Build history of the part. All positions in model axes, mm. A direction names the side the tool comes from. Give positions to 0.01 mm unless a question says otherwise; leave off trailing zeros. Order: outer loops, then holes, each group sorted by start corner. A loop starts at its lowest first (then second) coordinate and runs counter-clockwise, first axis right, second up. Notation, with made-up numbers: (-21.5, 28) - (-3.5, 28) arc R18 ccw to (-3.5, 52) - close; hole circle Ø4 at (-26, 36.5). An arc over 180 degrees is marked (long way). Answer in a Markdown table with one row per item.
```python
from build123d import *

# Parameters (mm, degrees)
F0_W      = 80
F0_H      = 40
F1_DEPTH  = 3
F2_R      = 3
F3_DEPTH  = 3
F5_D      = 2.5
F7_DEPTH  = 3
F9_D      = 3.25
F10_W     = 44.45
F10_H     = 19.05
F11_DEPTH = 6.001
F12_R     = 3
F13_R     = 1


# Not quite as in the source:
# - a pattern or mirror of a feature is missing from the dataset's text; its kind, count and spacing are read off the source's solid
# - a feature names something its author has since deleted; it is built from what else it names


with BuildPart() as f1:
    # F0 (on Top) → F1 (new body)
    with BuildSketch(Plane.XY):
        Rectangle(F0_W, F0_H)
    extrude(amount=F1_DEPTH)

    # F2 (on face) → F3 (join)
    with BuildSketch(Plane.XY.offset(3)):
        with Locations((-29, 11.5)):
            Circle(F2_R)
        with Locations((29, 11.5)):
            Circle(F2_R)
        with Locations((29, -11.5)):
            Circle(F2_R)
        with Locations((-29, -11.5)):
            Circle(F2_R)
    extrude(amount=F3_DEPTH)

    # F5 (through all)
    with Locations(Plane.XY.offset(6)):
        with Locations((-29, 11.5), (29, 11.5), (29, -11.5), (-29, -11.5)):
            Hole(F5_D / 2)

    # F6 (on face) → F7 (join)
    with BuildSketch(Plane(origin=(0, 0, 0), x_dir=(1, 0, 0), z_dir=(0, 0, -1))):
        with BuildLine():
            ThreePointArc((42.1213203436, 17.8786796564), (42.7716385975, 18.8519497029), (43, 20))
            ThreePointArc((43, 20), (41.1480502971, 22.7716385975), (37.8786796564, 22.1213203436))
            ThreePointArc((37.8786796564, 22.1213203436), (37.2283614025, 21.1480502971), (37, 20))
            Line((37, 20), (40, 20))
            Line((40, 20), (40, 17))
            ThreePointArc((40, 17), (41.1480502971, 17.2283614025), (42.1213203436, 17.8786796564))
        make_face()
        with BuildLine():
            ThreePointArc((37, 20), (37.2283614025, 21.1480502971), (37.8786796564, 22.1213203436))
            Line((37.8786796564, 22.1213203436), (35.7573593129, 20))
            Line((35.7573593129, 20), (37, 20))
        make_face()
        with BuildLine():
            Line((40, 15.7573593129), (42.1213203436, 17.8786796564))
            ThreePointArc((42.1213203436, 17.8786796564), (41.1480502971, 17.2283614025), (40, 17))
            Line((40, 17), (40, 15.7573593129))
        make_face()
        with BuildLine():
            Line((-37, 20), (-35.7573593129, 20))
            Line((-35.7573593129, 20), (-37.8786796564, 22.1213203436))
            ThreePointArc((-37.8786796564, 22.1213203436), (-37.2283614025, 21.1480502971), (-37, 20))
        make_face()
        with BuildLine():
            Line((42.1213203436, -17.8786796564), (40, -15.7573593129))
            Line((40, -15.7573593129), (40, -17))
            ThreePointArc((40, -17), (41.1480502971, -17.2283614025), (42.1213203436, -17.8786796564))
        make_face()
        with BuildLine():
            ThreePointArc((-37, 20), (-37.2283614025, 21.1480502971), (-37.8786796564, 22.1213203436))
            ThreePointArc((-37.8786796564, 22.1213203436), (-42.1213203436, 22.1213203436), (-42.1213203436, 17.8786796564))
            ThreePointArc((-42.1213203436, 17.8786796564), (-41.1480502971, 17.2283614025), (-40, 17))
            Line((-40, 17), (-40, 20))
            Line((-40, 20), (-37, 20))
        make_face()
        with BuildLine():
            ThreePointArc((43, -20), (42.7716385975, -18.8519497029), (42.1213203436, -17.8786796564))
            ThreePointArc((42.1213203436, -17.8786796564), (41.1480502971, -17.2283614025), (40, -17))
            Line((40, -17), (40, -20))
            Line((40, -20), (37, -20))
            ThreePointArc((37, -20), (37.2283614025, -21.1480502971), (37.8786796564, -22.1213203436))
            ThreePointArc((37.8786796564, -22.1213203436), (41.1480502971, -22.7716385975), (43, -20))
        make_face()
        with BuildLine():
            ThreePointArc((-40, 17), (-41.1480502971, 17.2283614025), (-42.1213203436, 17.8786796564))
            Line((-42.1213203436, 17.8786796564), (-40, 15.7573593129))
            Line((-40, 15.7573593129), (-40, 17))
        make_face()
        with BuildLine():
            ThreePointArc((37.8786796564, -22.1213203436), (37.2283614025, -21.1480502971), (37, -20))
            Line((37, -20), (35.7573593129, -20))
            Line((35.7573593129, -20), (37.8786796564, -22.1213203436))
        make_face()
        with BuildLine():
            Line((-40, -17), (-40, -15.7573593129))
            Line((-40, -15.7573593129), (-42.1213203436, -17.8786796564))
            ThreePointArc((-42.1213203436, -17.8786796564), (-41.1480502971, -17.2283614025), (-40, -17))
        make_face()
        with BuildLine():
            Line((-37.8786796564, -22.1213203436), (-35.7573593129, -20))
            Line((-35.7573593129, -20), (-37, -20))
            ThreePointArc((-37, -20), (-37.2283614025, -21.1480502971), (-37.8786796564, -22.1213203436))
        make_face()
        with BuildLine():
            ThreePointArc((-40, -17), (-41.1480502971, -17.2283614025), (-42.1213203436, -17.8786796564))
            ThreePointArc((-42.1213203436, -17.8786796564), (-42.1213203436, -22.1213203436), (-37.8786796564, -22.1213203436))
            ThreePointArc((-37.8786796564, -22.1213203436), (-37.2283614025, -21.1480502971), (-37, -20))
            Line((-37, -20), (-40, -20))
            Line((-40, -20), (-40, -17))
        make_face()
    extrude(amount=-F7_DEPTH)

    # F9 (through all)
    with Locations(Plane(origin=(0, 0, 0), x_dir=(1, 0, 0), z_dir=(0, 0, -1))):
        with Locations((-40, 20), (-40, -20), (40, -20)):
            f9 = Hole(F9_D / 2)

    # F9_copies: F9 across plane
    add(f9.mirror(Plane(origin=(0, 0, 0), x_dir=(0, 0, 1), z_dir=(1, 0, 0))), mode=Mode.SUBTRACT)

    # F10 (on face) → F11 (cut, through all)
    with BuildSketch(Plane(origin=(0, 0, 0), x_dir=(1, 0, 0), z_dir=(0, 0, -1))):
        Rectangle(F10_W, F10_H)
    extrude(amount=-F11_DEPTH, mode=Mode.SUBTRACT)

    # F12
    f12_edges = [f1.edges().sort_by_distance(p)[0] for p in [
        (-22.225, 9.525, 1.5),
        (22.225, -9.525, 1.5),
        (-22.225, -9.525, 1.5),
        (22.225, 9.525, 1.5),
    ]]
    fillet(f12_edges, radius=F12_R)

    # F13
    f13_edges = [f1.edges().sort_by_distance(p)[0] for p in [
        (40, 15.757359, 1.5),
        (-40, 15.757359, 1.5),
        (40, -15.757359, 1.5),
        (-40, -15.757359, 1.5),
    ]]
    fillet(f13_edges, radius=F13_R)


solid = f1.part
```
1. Drop flat-ended pins along their axis: P1, Ø3, axis at x = -18, y = 7, coming from the -Z side; P2, Ø1, axis at x = -24.5, z = 1.5, coming from the +Y side; P3, Ø0.9, axis at x = 13, z = 1, coming from the -Y side; P4, Ø1.5, axis at y = 0.5, z = 1.5, coming from the +X side. Give the stop position or say it passes through.
Check result:
| item | result |
|---|---|
| P1 | passes through |
| P2 | stops at y = 20 |
| P3 | stops at y = -20 |
| P4 | stops at x = 40 |
2. Probe line 1 (Y direction, x = 29, z = 2.95); line 2 (Y direction, x = 29, z = 3.75); line 3 (Y direction, x = 0.5, z = 2.35) (3 decimals). List the from-to ranges inside material, lowest first.
Check result:
| item | result |
|---|---|
| line 1 | y = -20 to -12.75, -10.25 to 10.25, 12.75 to 20 |
| line 2 | y = -14.5 to -12.75, -10.25 to -8.5, 8.5 to 10.25, 12.75 to 14.5 |
| line 3 | y = -20 to -9.525, 9.525 to 20 |
3. Cut at B-B on y = 11.5. Write the cut outline in (x, z), and give its area (3 significant figures).
Check result:
| item | result |
|---|---|
| outline | (-40, 0) - (-30.25, 0) - (-30.25, 6) - (-32, 6) - (-32, 3) - (-40, 3) - close; (-27.75, 0) - (27.75, 0) - (27.75, 6) - (26, 6) - (26, 3) - (-26, 3) - (-26, 6) - (-27.75, 6) - close; (30.25, 0) - (40, 0) - (40, 3) - (32, 3) - (32, 6) - (30.25, 6) - close |
| area | 246 mm² |
4. Which spindle directions (+Z, -Z, +X, -X, +Y, -Y) get a long thin tool onto all of the face, cutting with end or side? Do faces 4 (the face through (40, 0, 1)), 5 (the face through (21.32, 8.67, 1.52)), 6 (the face through (-1, 10, 3)). Say none if no direction does.
Check result:
| item | result |
|---|---|
| face 4 | +Z, -Z, +X |
| face 5 | +Z, -Z |
| face 6 | +Z |
5. Cut at D-D on y = -5.5. Write the cut outline in (x, z) (3 decimals).
Check result:
| item | result |
|---|---|
| outline | (-40, 0) - (-22.225, 0) - (-22.225, 3) - (-40, 3) - close; (22.225, 0) - (40, 0) - (40, 3) - (22.225, 3) - close |
6. Cut at C-C on x = 29. Write the cut outline in (y, z).
Check result:
| item | result |
|---|---|
| outline | (-20, 0) - (-12.75, 0) - (-12.75, 6) - (-14.5, 6) - (-14.5, 3) - (-20, 3) - close; (-10.25, 0) - (10.25, 0) - (10.25, 6) - (8.5, 6) - (8.5, 3) - (-8.5, 3) - (-8.5, 6) - (-10.25, 6) - close; (12.75, 0) - (20, 0) - (20, 3) - (14.5, 3) - (14.5, 6) - (12.75, 6) - close |
7. Cut at A-A on z = 4.7. Write the cut outline in (x, y).
Check result:
| item | result |
|---|---|
| outline | circle Ø6 at (-29, -11.5); circle Ø6 at (-29, 11.5); circle Ø6 at (29, -11.5); circle Ø6 at (29, 11.5); hole circle Ø2.5 at (-29, -11.5); hole circle Ø2.5 at (-29, 11.5); hole circle Ø2.5 at (29, -11.5); hole circle Ø2.5 at (29, 11.5) |
8. Two-plate mould, pull along X, no slides. Class faces 1 (the face through (29, -13, 6)), 2 (the face through (-29.672, -10.446, 2.958)), 3 (the face through (41.19, -16.95, 1.48)): +X half, -X half, draft (parallel to the pull), parting line (faces both ways), or undercut.
Check result:
| item | result |
|---|---|
| face 1 | draft |
| face 2 | undercut |
| face 3 | +X half |
